Work out the finished part from the listing and answer in its coordinate system (mm). A direction names the side the tool comes from. Give positions to 0.01 mm unless a question says otherwise; leave off trailing zeros. Write each loop counter-clockwise with the first axis right and the second up, starting at its lowest first coordinate (ties: lowest second). Pieces come first, ordered by that corner, then holes.
1) Given pin 1 Ø1.5 at (x, y) = (-48, -7.5) entering from -Z; pin 2 Ø5 at (x, z) = (40.5, 48) entering from -Y; pin 3 Ø1 at (y, z) = (-5, -34) entering from -X, each flat-ended and moving along its own axis, determine where each tip first touches the part or whether it passes through.
2) Find section C-C (y = -7.5). Determine the outline of the cut face in (x, z).
3) A tool of negligible diameter and unlimited length cuts with its end or side. For faces 1 (the face through (58, -3.048, 13)), 2 (the face through (-50.9, -1.5, -32.45)), from which of +Z, -Z, +X, -X, +Y, -Y can it reach the whole face along a straight path? Write none if from no direction.
4) Straight lines are drawn through the part: probe 1 along Z at (x, y) = (1, -8.25); probe 2 along X at (y, z) = (-6, 0); probe 3 along Y at (x, z) = (-43, -42). For each, find the intervals that lie inside material, in ascending order.
5) Find section B-B (z = 0). Determine the outline of the cut face in (x, y) (1 decimal).
6) Determine the mould class of faces 3 (the face through (-54.09, -5.33, 7.1)), 4 (the face through (56.07, -6.92, 12.45)), 5 (the face through (21, -9.271, 51)) for opening direction Z: pulls with the +Z half, pulls with the -Z half, needs draft (parallel to the pull), parting line crosses it, or undercut.
7) Find section A-A (x = 0). Determine the outline of the cut face in (y, z) (1 decimal).
```python
from build123d import *

# Parameters (mm, degrees)
CHAMFER1_SIZE = 1.27
FILLET1_R     = 1.5875


with BuildPart() as part:
    # Sketch1 → Revolve1 (revolve)
    with BuildSketch(Plane.XY, mode=Mode.PRIVATE) as revolve1_sk:
        Polygon((-54.55285, 0), (-54.55285, -9.271), (-57.43575, -9.271), (-57.43575, -3.048), (-60.3631, -3.048), (-60.3631, 0), align=None)
    revolve(revolve1_sk.sketch.rotate(Axis((0, 0, 0), (0, 1, 0)), 270), axis=Axis((0, 0, 0), (0, 1, 0)))

    # Chamfer1
    chamfer1_edges = [part.edges().sort_by_distance(p)[0] for p in [
        (0, 0, 54.55285),
    ]]
    chamfer(chamfer1_edges, length=CHAMFER1_SIZE)

    # Fillet1
    fillet1_edges = [part.edges().sort_by_distance(p)[0] for p in [
        (0, -3.048, 57.43575),
    ]]
    fillet(fillet1_edges, radius=FILLET1_R)


solid = part.part
```
Results:
1. pin 1: stops at z = -32.65
1. pin 2: stops at y = -3.05
1. pin 3: stops at x = -46.65
2. outline: circle Ø114.87 at (0, 0); hole circle Ø109.11 at (0, 0)
3. face 1: -Y
3. face 2: +Y, -Y
4. probe 1: z = -57.43 to -54.54, 54.54 to 57.43
4. probe 2: x = -57.44 to -54.55, 54.55 to 57.44
4. probe 3: y = -3.05 to 0
5. outline: (-60.4, -3) - (-59, -3) arc R1.6 cw to (-57.4, -4.6) - (-57.4, -9.3) - (-54.6, -9.3) - (-54.6, -1.3) - (-55.8, 0) - (-60.4, 0) - close; (54.6, -9.3) - (57.4, -9.3) - (57.4, -4.6) arc R1.6 cw to (59, -3) - (60.4, -3) - (60.4, 0) - (55.8, 0) - (54.6, -1.3) - close
6. face 3: undercut
6. face 4: parting line crosses it
6. face 5: needs draft
7. outline: (-9.3, -57.4) - (-4.6, -57.4) arc R1.6 cw to (-3, -59) - (-3, -60.4) - (0, -60.4) - (0, -55.8) - (-1.3, -54.6) - (-9.3, -54.6) - close; (-9.3, 54.6) - (-1.3, 54.6) - (0, 55.8) - (0, 60.4) - (-3, 60.4) - (-3, 59) arc R1.6 cw to (-4.6, 57.4) - (-9.3, 57.4) - close
